```python
from build123d import *

# Parameters (mm, degrees)
SKETCH1_R                 = 13.85
BOSS_EXTRUDE1_DEPTH       = 19
SKETCH2_R                 = 2.5
BOSS_EXTRUDE2_DEPTH       = 14
M3X0_5_TAPPED_HOLE1_D     = 2.5
M3X0_5_TAPPED_HOLE1_DEPTH = 7.5
M3X0_5_TAPPED_HOLE1_TIP   = 0.751075774
BOSS_EXTRUDE3_START       = -0.449533
BOSS_EXTRUDE3_DEPTH       = 4.449533


with BuildPart() as part:
    # Sketch1 → Boss-Extrude1 (new body)
    with BuildSketch(Plane(origin=(0, 0, 0), x_dir=(1, 0, 0), z_dir=(0, 1, 0))):
        Circle(SKETCH1_R)
    extrude(amount=BOSS_EXTRUDE1_DEPTH)

    # Sketch2 → Boss-Extrude2 (add)
    with BuildSketch(Plane(origin=(0, 19, 0), x_dir=(1, 0, 0), z_dir=(0, 1, 0))):
        Circle(SKETCH2_R)
    extrude(amount=BOSS_EXTRUDE2_DEPTH)

    # M3x0.5 Tapped Hole1
    with Locations(Plane(origin=(0, 0, 0), x_dir=(-1, 0, 0), z_dir=(0, -1, 0))):
        with Locations((0, -8), (9.5, 0), (0, 8), (-9.5, 0)):
            Hole(M3X0_5_TAPPED_HOLE1_D / 2, depth=M3X0_5_TAPPED_HOLE1_DEPTH)
            with Locations((0, 0, -(M3X0_5_TAPPED_HOLE1_DEPTH + M3X0_5_TAPPED_HOLE1_TIP / 2))):  # 118° drill point
                Cone(0, M3X0_5_TAPPED_HOLE1_D / 2, M3X0_5_TAPPED_HOLE1_TIP, mode=Mode.SUBTRACT)

    # Sketch7 → Boss-Extrude3 (add)
    with BuildSketch(Plane(origin=(9.793428919, 0, 9.793428919), x_dir=(0.707106781, 0, -0.707106781), z_dir=(0.707106781, 0, 0.707106781)).offset(BOSS_EXTRUDE3_START)):
        with BuildLine():
            Line((-2.5, 2), (2.5, 2))
            ThreePointArc((2.5, 2), (3.5, 1), (2.5, 0))
            Line((2.5, 0), (-2.5, 0))
            ThreePointArc((-2.5, 0), (-3.5, 1), (-2.5, 2))
        make_face()
    extrude(amount=BOSS_EXTRUDE3_DEPTH)


solid = part.part
```
Input: part model. Units: mm. Frame: model coordinates. A direction names the side the tool comes from. Coordinates: 2 decimals unless noted, no trailing zeros. Write each loop counter-clockwise with the first axis right and the second up, starting at its lowest first coordinate (ties: lowest second). Pieces come first, ordered by that corner, then holes. Notation, with made-up numbers: (51, -2.5) -> (67, -2.5) arc R25 cw to (67, 16.5) -> close; hole circle Ø3 at (17, 21.5). An arc over 180 degrees is marked (long way). Answer as a JSON object with one key per item and string values.
1. Section A-A on y = 7. Return the cut outline in (x, z).
Result set:
{"outline": "circle Ø27.7 at (0, 0); hole circle Ø2.5 at (-9.5, 0); hole circle Ø2.5 at (0, -8); hole circle Ø2.5 at (0, 8); hole circle Ø2.5 at (9.5, 0)"}
2. Mould query, pull axis Z, two halves, no side actions, for faces 1 (the face through (12.657, 1.014, 12.587)), 2 (the face through (-0.54, 25.9, 2.44)), 3 (the face through (8.25, 3.8, -0.05)), 4 (the face through (11, 2, 11)). Classes: released by +Z, released by -Z, zero draft, split by the parting line, or undercut.
Result set:
{"face 1": "released by +Z", "face 2": "split by the parting line", "face 3": "undercut", "face 4": "zero draft"}
3. Section B-B on y = 22. Return the cut outline in (x, z), then the cut area to 3 significant figures.
Result set:
{"outline": "circle Ø5 at (0, 0)", "area": "19.6 mm2"}
4. First-contact query: P1, Ø5, axis at x = 12.5, z = 10, coming from the +Y side; P2, Ø3, axis at y = 6, z = 5, coming from the -X side; P3, Ø2, axis at x = 9.5, z = 0, coming from the -Y side; P4, Ø4, axis at x = 0, z = 8, coming from the -Y side. Flat tips, straight axial feed; report the tip coordinate or a pass-through.
Result set:
{"P1": "stops at y = 19", "P2": "stops at x = -13.4", "P3": "stops at y = 7.65", "P4": "stops at y = 0"}
5. Material intervals for line 1 (Z direction, x = 0, y = 2.5); line 2 (Y direction, x = -6, z = 8.75); line 3 (Y direction, x = 11, z = 10.25), sorted ascending. Write a range as from..to.
Result set:
{"line 1": "z = -13.85..-9.25, -6.75..6.75, 9.25..13.85", "line 2": "y = 0..19", "line 3": "y = 0..2"}
6. Section D-D on x = -11.5. Return the cut outline in (y, z), then the cut area to 3 significant figures.
Result set:
{"outline": "(0, -7.72) -> (19, -7.72) -> (19, 7.72) -> (0, 7.72) -> close", "area": "293 mm2"}
7. Access query for faces 5 (the face through (13.5, 1.02, 8.55)), 6 (the face through (8.55, 0.98, 13.5)), 7 (the face through (-0.27, 3.8, -6.78)). Directions: +Z, -Z, +X, -X, +Y, -Y. A direction counts if a zero-diameter tool reaches every point of the face in a straight line with its end or side. Return the directions, or none.
Result set:
{"face 5": "+X", "face 6": "+Z", "face 7": "-Y"}
8. Section C-C on z = -5.75. Return the cut outline in (x, y).
Result set:
{"outline": "(-12.6, 0) -> (12.6, 0) -> (12.6, 19) -> (-12.6, 19) -> close"}
